```python
from build123d import *

# Parameters (mm, degrees)
EXTRUDE_1_DEPTH     = 5
CUT_EXTRUDE_1_DEPTH = 1.5
SKETCH_2_R          = 4
EXTRUDE_2_DEPTH     = 16
CUT_EXTRUDE_2_DEPTH = 5
CHAMFER_2_SIZE      = 1


with BuildPart() as part:
    # Эскиз1 → Бобышка-Вытянуть1 (new body, symmetric)
    with BuildSketch(Plane.XY):
        Polygon((9.75, 0), (-9.75, 0), (-9.75, 4), (-5, 4), (-5, 5.5), (5, 5.5), (5, 4), (9.75, 4), align=None)
    extrude(amount=EXTRUDE_1_DEPTH, both=True)

    # Эскиз3 → Вырез-Вытянуть1 (cut)
    with BuildSketch(Plane(origin=(0, 5.5, 0), x_dir=(1, 0, 0), z_dir=(0, 1, 0))):
        with BuildLine():
            Line((-5, 0), (-5, 5))
            Line((-5, 5), (0, 5))
            ThreePointArc((0, 5), (-3.535533906, 3.535533906), (-5, 0))
        make_face()
        with BuildLine():
            Line((0, -5), (5, -5))
            Line((5, -5), (5, 0))
            ThreePointArc((5, 0), (3.535533906, -3.535533906), (0, -5))
        make_face()
    extrude(amount=-CUT_EXTRUDE_1_DEPTH, mode=Mode.SUBTRACT)

    # Эскиз2 → Бобышка-Вытянуть2 (add)
    with BuildSketch(Plane(origin=(0, 5.5, 0), x_dir=(1, 0, 0), z_dir=(0, 1, 0))):
        with Locations(Location((0, 0, 0), (0, 0, 270))):  # turned: the seam where the file's is
            Circle(SKETCH_2_R)
    extrude(amount=EXTRUDE_2_DEPTH)

    # Эскиз4 → Вырез-Вытянуть2 (cut, through all)
    with BuildSketch(Plane(origin=(0, 4, 0), x_dir=(1, 0, 0), z_dir=(0, 1, 0))):
        with BuildLine():
            Line((-8.370334521, 5), (-9.75, 5))
            Line((-9.75, 5), (-9.75, 0))
            ThreePointArc((-9.75, 0), (-9.398756875, 2.59342808), (-8.370334521, 5))
        make_face()
        with BuildLine():
            Line((8.370334521, -5), (9.75, -5))
            Line((9.75, -5), (9.75, 0))
            ThreePointArc((9.75, 0), (9.398756875, -2.59342808), (8.370334521, -5))
        make_face()
    extrude(amount=-CUT_EXTRUDE_2_DEPTH, mode=Mode.SUBTRACT)

    # Вырез-По траектории1: sweep along a path in Эскиз6
    with BuildLine(Plane.XZ) as sweep_1_path:
        Line((0, -9.75), (9.75, -9.75))
        Line((9.75, -9.75), (9.75, 0))
        ThreePointArc((9.75, 0), (6.894291117, 6.894291117), (0, 9.75))
        Line((0, 9.75), (-9.75, 9.75))
        Line((-9.75, 9.75), (-9.75, 0))
        ThreePointArc((-9.75, 0), (-6.894291117, -6.894291117), (0, -9.75))
    # Эскиз5 → Вырез-По траектории1 (sweep, cut)
    with BuildSketch(Plane.XY.offset(5)):
        Polygon((-9.75, 2.5), (-5.8, 0), (-9.75, 0), align=None)
    sweep(path=sweep_1_path.line, transition=Transition.RIGHT, mode=Mode.SUBTRACT)

    # Фаска2
    chamfer_2_edges = [part.edges().sort_by_distance(p)[0] for p in [
        (0, 21.5, -4),
    ]]
    chamfer(chamfer_2_edges, length=CHAMFER_2_SIZE)


solid = part.part
```
Verification items for the finished model (mm, model axes). A direction names the side the tool comes from. Coordinates: 2 decimals unless noted, no trailing zeros. Loops run counter-clockwise (first coordinate to the right, second up) from the corner with the lowest first, then second, coordinate; pieces in that order, holes last. Notation, with made-up numbers: (17, 53.5) - (33, 53.5) arc R28 ccw to (33, 91.5) - close; hole circle Ø10 at (66, -16). An arc over 180 degrees is marked (long way). Answer as a JSON object with one key per item and string values.
(1) Cross-section at B-B, the plane y = 17.5. Record the boundary of the cut face in (x, z).
Response:
{"outline": "circle Ø8 at (0, 0)"}
(2) Go/stop test with flat-tipped pins: pin 1 Ø8 at (x, y) = (0, 14.5) entering from +Z; pin 2 Ø3 at (x, z) = (5.5, 1) entering from +Y; pin 3 Ø1 at (x, y) = (-8, 5.5) entering from -Z; pin 4 Ø3 at (y, z) = (17, -2.5) entering from +X. Record where each tip stops, or that it passes through.
Response:
{"pin 1": "stops at z = 4", "pin 2": "stops at y = 5.5", "pin 3": "passes through", "pin 4": "stops at x = 3.87"}
(3) Scan lines: line 1 along X through (y, z) = (14, -1.5); line 2 along X through (y, z) = (5.75, 3); line 3 along Y through (x, z) = (5.5, -4). Record each from-to range of solid material in increasing order.
Response:
{"line 1": "x = -3.71 to 3.71", "line 2": "x = -2.65 to 2.65", "line 3": "y = 0 to 4"}
(4) Cross-section at A-A, the plane y = 2.75. Record the boundary of the cut face in (x, z), then the cut area to 3 significant figures.
Response:
{"outline": "(-9.75, 0) arc R9.75 ccw to (-8.37, -5) - (9.75, -5) - (9.75, 0) arc R9.75 ccw to (8.37, 5) - (-9.75, 5) - close", "area": "191 mm²"}
(5) Access from +Z, -Z, +X, -X, +Y, -Y to the whole of each face (thin tool, end or side, straight path). Record for faces 1 (the cylindrical face through (-3, 5, -4)), 2 (the cylindrical face through (4, 5, 3)), 3 (the flat face through (5, 5, -2)), 4 (the flat face through (-0.1, 5.5, 4.5)), 5 (the flat face through (-5, 5, 3)).
Response:
{"face 1": "-Z, -X, +Y", "face 2": "+Z, +X, +Y", "face 3": "+Z, -Z, +X, +Y", "face 4": "+Y", "face 5": "+Z, -Z, -X, +Y"}
